```python
from build123d import *

# Parameters (mm, degrees)
BOSS_EXTRUDE1_DEPTH         = 3.175
M3_CLEARANCE_HOLE1_D        = 3.6
F_1_4_CLEARANCE_HOLE1_D     = 7.14248
CUT_EXTRUDE1_DEPTH          = 640.11012417
F_8_CLEARANCE_HOLE1_D       = 4.9149
SKETCH15_R                  = 1.55
CUT_EXTRUDE2_DEPTH          = 640.11012417
SKETCH16_R                  = 3.3782
CUT_EXTRUDE3_DEPTH          = 640.11012417
FILLET1_R                   = 1
CUT_EXTRUDE4_DEPTH          = 640.088878697
FILLET2_R                   = 1.5
F_13_0_185_DIAMETER_HOLE1_D = 4.699
F_1_4_CLEARANCE_HOLE2_D     = 6.7564
SKETCH23_W                  = 10
SKETCH23_H                  = 17
CUT_EXTRUDE5_DEPTH          = 640.088878697
FILLET3_R                   = 2
F_5_0MM_DOWEL_HOLE1_D       = 5


with BuildPart() as part:
    # Sketch1 → Boss-Extrude1 (new, symmetric)
    with BuildSketch(Plane(origin=(0, 0, 0), x_dir=(1, 0, 0), z_dir=(0, 1, 0))):
        Polygon((0, -94.3735), (0, 94.3735), (-621.526239041, 148.75), (-621.526239041, -148.75), align=None)
    extrude(amount=BOSS_EXTRUDE1_DEPTH, both=True)

    # M3 Clearance Hole1 (through all)
    with Locations(Plane(origin=(0, 3.175, 0), x_dir=(1, 0, 0), z_dir=(0, 1, 0))):
        with Locations((-379.222, 34.29), (-384.81, 34.29), (-384.81, -34.29)):
            Hole(M3_CLEARANCE_HOLE1_D / 2)

    # 1/4 Clearance Hole1 (through all)
    with Locations(Plane(origin=(0, 3.175, 0), x_dir=(1, 0, 0), z_dir=(0, 1, 0))):
        with Locations((-187.837254031, 59.752653333), (-42.931947364, 59.752653333), (-42.931947364, -59.752653333), (-187.837254031, -59.752653333)):
            Hole(F_1_4_CLEARANCE_HOLE1_D / 2)

    # Sketch12 → Cut-Extrude1 (cut, through all)
    with BuildSketch(Plane(origin=(0, 3.175, 0), x_dir=(1, 0, 0), z_dir=(0, 1, 0))):
        with BuildLine():
            Line((-380.84125, -33.6169), (-380.84125, -34.0868))
            ThreePointArc((-380.84125, -34.0868), (-380.85395, -34.29), (-380.84125, -34.4932))
            Line((-380.84125, -34.4932), (-380.84125, -34.9631))
            ThreePointArc((-380.84125, -34.9631), (-379.222, -36.58235), (-377.60275, -34.9631))
            Line((-377.60275, -34.9631), (-377.60275, -34.4932))
            ThreePointArc((-377.60275, -34.4932), (-377.59005, -34.29), (-377.60275, -34.0868))
            Line((-377.60275, -34.0868), (-377.60275, -33.6169))
            ThreePointArc((-377.60275, -33.6169), (-379.222, -31.99765), (-380.84125, -33.6169))
        make_face()
    extrude(amount=-CUT_EXTRUDE1_DEPTH, mode=Mode.SUBTRACT)

    # #8 Clearance Hole1 (through all)
    with Locations(Plane(origin=(0, 3.175, 0), x_dir=(1, 0, 0), z_dir=(0, 1, 0))):
        with Locations((-506.81796477, -78.064272283), (-506.81796477, -103.464272283), (-541.198220891, -112.444528404), (-532.21796477, -78.064272283), (-479.392709852, -78.064272283), (-479.392709852, -103.464272283), (-453.992709852, -78.064272283), (-453.992709852, -103.464272283), (-453.992709852, 78.064272283), (-453.992709852, 103.464272283), (-479.392709852, 78.064272283), (-479.392709852, 103.464272283), (-541.198220891, 112.444528404), (-532.21796477, 78.064272283), (-506.81796477, 103.464272283), (-506.81796477, 78.064272283)):
            Hole(F_8_CLEARANCE_HOLE1_D / 2)

    # Sketch15 → Cut-Extrude2 (cut, through all)
    with BuildSketch(Plane(origin=(0, 3.175, 0), x_dir=(1, 0, 0), z_dir=(0, 1, 0))):
        with Locations(Location((-295.918163181, -81.916960017, 0), (0, 0, 270))):
            Circle(SKETCH15_R)
        with Locations(Location((-364.1575, -87.887128395, 0), (0, 0, 270))):
            Circle(SKETCH15_R)
    extrude(amount=-CUT_EXTRUDE2_DEPTH, mode=Mode.SUBTRACT)

    # Sketch16 → Cut-Extrude3 (cut, through all)
    with BuildSketch(Plane(origin=(0, 3.175, 0), x_dir=(1, 0, 0), z_dir=(0, 1, 0))):
        with Locations(Location((-609.6000104, -121.650317511, 0), (0, 0, 270))):
            Circle(SKETCH16_R)
        with Locations(Location((-609.6000104, -86.943080709, 0), (0, 0, 270))):
            Circle(SKETCH16_R)
        with Locations(Location((-609.6000104, 86.943080709, 0), (0, 0, 270))):
            Circle(SKETCH16_R)
        with Locations(Location((-609.6000104, 121.650317511, 0), (0, 0, 270))):
            Circle(SKETCH16_R)
    extrude(amount=-CUT_EXTRUDE3_DEPTH, mode=Mode.SUBTRACT)

    # Fillet1
    fillet1_edges = [part.edges().sort_by_distance(p)[0] for p in [
        (-621.526239041, 0, 148.75),
        (-621.526239041, 0, -148.75),
    ]]
    fillet(fillet1_edges, radius=FILLET1_R)

    # Sketch17 → Cut-Extrude4 (cut, through all)
    with BuildSketch(Plane(origin=(0, 3.175, 0), x_dir=(1, 0, 0), z_dir=(0, 1, 0))):
        Polygon((-3, 94.635965991), (-3, 59.635965991), (0, 59.635965991), (0, 94.3735), align=None)
    cut_extrude4 = extrude(amount=-CUT_EXTRUDE4_DEPTH, mode=Mode.SUBTRACT)

    # Mirror1: Cut-Extrude4 across plane
    add(cut_extrude4.mirror(Plane.XY), mode=Mode.SUBTRACT)

    # Fillet2
    fillet2_edges = [part.edges().sort_by_distance(p)[0] for p in [
        (0, 0, -59.635965991),
        (-3, 0, -59.635965991),
        (-3, 0, -94.635965991),
        (0, 0, 59.635965991),
        (-3, 0, 59.635965991),
        (-3, 0, 94.635965991),
    ]]
    fillet(fillet2_edges, radius=FILLET2_R - 0.0001)  # a hair under: the kernel refuses the full size

    # #13 (0.185) Diameter Hole1 (through all)
    with Locations(Plane(origin=(0, 3.175, 0), x_dir=(1, 0, 0), z_dir=(0, 1, 0))):
        with Locations((-354.44558465, 73.187743603), (-304.635849746, 68.829956465)):
            Hole(F_13_0_185_DIAMETER_HOLE1_D / 2)

    # 1/4 Clearance Hole2 (through all)
    with Locations(Plane(origin=(0, 3.175, 0), x_dir=(1, 0, 0), z_dir=(0, 1, 0))):
        with Locations((-14.732, 88.469940408), (-14.0462, -87.453940528), (-303.7332, 0)):
            Hole(F_1_4_CLEARANCE_HOLE2_D / 2)

    # Sketch23 → Cut-Extrude5 (cut, through all)
    with BuildSketch(Plane(origin=(0, 3.175, 0), x_dir=(1, 0, 0), z_dir=(0, 1, 0))):
        with Locations((-616.526239041, 140.158691499)):
            Rectangle(SKETCH23_W, SKETCH23_H)
        with Locations((-616.526239041, -140.158691499)):
            Rectangle(SKETCH23_W, SKETCH23_H)
    extrude(amount=-CUT_EXTRUDE5_DEPTH, mode=Mode.SUBTRACT)

    # Fillet3
    fillet3_edges = [part.edges().sort_by_distance(p)[0] for p in [
        (-611.526239041, 0, -147.875113365),
        (-621.526239041, 0, -131.658691499),
        (-611.526239041, 0, -131.658691499),
        (-611.526239041, 0, 147.875113365),
        (-611.526239041, 0, 131.658691499),
        (-621.526239041, 0, 131.658691499),
    ]]
    fillet(fillet3_edges, radius=FILLET3_R)

    # Ø5.0mm Dowel Hole1 (through all)
    with Locations(Plane(origin=(0, 3.175, 0), x_dir=(1, 0, 0), z_dir=(0, 1, 0))):
        with Locations((-163.962100698, -41.275), (-66.807100698, -41.275)):
            Hole(F_5_0MM_DOWEL_HOLE1_D / 2)


solid = part.part
```
Check sheet for the modelled part. Datum: model origin and axes. Units: mm. Give positions to 0.01 mm unless a question says otherwise; leave off trailing zeros. Loops run counter-clockwise (first coordinate to the right, second up) from the corner with the lowest first, then second, coordinate; pieces in that order, holes last. Notation, with made-up numbers: M -38.75,10.5 L 17.25,10.5 A20 ccw 17.25,46.5 Z; hole C -18.5,89 d4. An arc over 180 degrees is marked long. Answer as CSV lines item,"result".
Item 1: Sectioned sample at C-C, the plane x = -557.5. Enter the section's corners in (y, z) (3 decimals).
Reply:
outline,"M -3.175,-143.148 L 3.175,-143.148 L 3.175,143.148 L -3.175,143.148 Z"
Item 2: Depth check by flat-ended pin: pin 1 Ø6 at (x, z) = (-66.81, 41.28) entering from +Y (3 decimals); pin 2 Ø3 at (y, z) = (1, 71) entering from +X; pin 3 Ø3 at (x, y) = (-498, 1) entering from +Z. Enter the tip coordinate at first touch or a pass-through.
Reply:
pin 1,"y = 3.175"
pin 2,"x = -3"
pin 3,"z = 138.07"
Item 3: Sectioned sample at B-B, the plane y = -0.25. State how many separate pieces and enclosed holes the cut face has, then the cut area to 3 significant figures.
Reply:
separate pieces,"1"
enclosed holes,"37"
area,"150,000 mm^2"
Item 4: Scan lines: L1, parallel to X at y = 1.5, z = -78.5; L2, parallel to X at y = 3, z = 87; L3, parallel to X at y = 0.75, z = 59. Record each from-to range of solid material in increasing order.
Reply:
L1,"-621.53 to -534.64, -529.8 to -509.24, -504.4 to -481.81, -476.97 to -456.41, -451.57 to -3"
L2,"-621.53 to -612.98, -606.22 to -365.43, -362.89 to -17.39, -10.7 to -3"
L3,"-621.53 to -191.33, -184.35 to -46.42, -39.44 to -0.27"
Item 5: Sectioned sample at A-A, the plane x = -135. Enter the section's corners in (y, z) (3 decimals).
Reply:
outline,"M -3.175,-106.184 L 3.175,-106.184 L 3.175,106.184 L -3.175,106.184 Z"
